from build123d import *

# Parameters (mm, degrees)
F0_W     = 32
F0_H     = 32
F1_DEPTH = 20
F2_T     = -2.5
F3_R     = 4
F4_DEPTH = 4


with BuildPart() as f1:
    # F0 (on Top) → F1 (new body)
    with BuildSketch(Plane.XY):
        with Locations((-40.726009, 25.983708)):
            Rectangle(F0_W, F0_H)
    extrude(amount=F1_DEPTH)

    # F2
    f2_openings = [f1.faces().sort_by_distance(p)[0] for p in [
        (-40.726009, 25.983708, 0),
    ]]
    offset(amount=F2_T, openings=f2_openings)

    # F3 (on face) → F4 (join)
    with BuildSketch(Plane.XY.offset(20)):
        with Locations((-49.358711, 33.123519)):
            Circle(F3_R)
        with Locations((-49.358711, 17.261552)):
            Circle(F3_R)
        with Locations((-32.003853, 17.261552)):
            Circle(F3_R)
        with Locations((-32.003853, 33.123519)):
            Circle(F3_R)
    extrude(amount=F4_DEPTH)


solid = f1.part
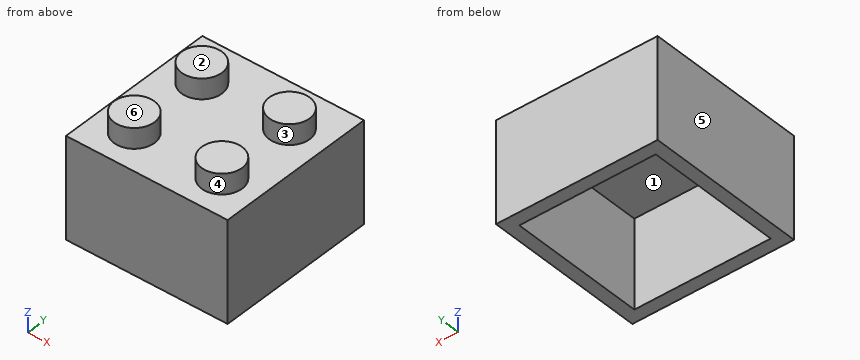
Can you work these out from the model? Positions are in its coordinate system, mm. Face numbers are marked on the shaded views. A direction names the side the tool comes from. Give positions to 0.01 mm unless a question says otherwise; leave off trailing zeros. Loops run counter-clockwise (first coordinate to the right, second up) from the corner with the lowest first, then second, coordinate; pieces in that order, holes last. Notation, with made-up numbers: M 13.25,-17.5 L 31.25,-17.5 A15 cw 31.25,4.5 Z; hole C -32.5,44.5 d11. An arc over 180 degrees is marked long. One line per item, written item: value. Start each with the question number.
1) On a 3-axis mill with a long thin cutter (end or side, diameter ignored), from which of +Z, -Z, +X, -X, +Y, -Y can I reach the whole of each face in a straight line? I mean the marked faces 1, 2 and 3. Say none if no direction works.
2) Thinking about a two-plate mould opening in X: for the marked faces 4, 5 and 6, which applies, +X half, -X half, draft (parallel to the pull), parting line (faces both ways), or undercut?
3) I'm going to push flat-ended pins straight in: pin 1 (1.5 mm diameter, centred on x = -42.5, y = 17.5, fed in from -Z); pin 2 (3 mm diameter, centred on x = -36.5, y = 21.5, fed in from +Z). Where does each tip first touch, or does it pass through?
4) If we section it at A-A, the plane z = 10.5: Write out the boundary of the cut face in (x, y), and give its area (3 significant figures).
5) If we section it at B-B, the plane x = -41: Write out the boundary of the cut face in (y, z).
6) If I drill on line 1 (X direction, y = 16, z = 7.75); line 2 (Y direction, x = -40.5, z = 9.75); line 3 (Z direction, x = -43, y = 40), over which ranges is the centre line in solid material (lowest first)? Write a range as [from, to].
7) If we section it at D-D, the plane x = -32.5: Write out the boundary of the cut face in (y, z), and give its area (3 significant figures).
8) If we section it at C-C, the plane y = 27: Write out the boundary of the cut face in (x, z).
Completed:
1. face 1: -Z
1. face 2: +Z, +X, -X, +Y, -Y
1. face 3: +Z
2. face 4: undercut
2. face 5: -X half
2. face 6: draft
3. pin 1: stops at z = 17.5
3. pin 2: stops at z = 20
4. outline: M -56.73,9.98 L -24.73,9.98 L -24.73,41.98 L -56.73,41.98 Z; hole M -54.23,12.48 L -27.23,12.48 L -27.23,39.48 L -54.23,39.48 Z
4. area: 295 mm^2
5. outline: M 9.98,0 L 12.48,0 L 12.48,17.5 L 39.48,17.5 L 39.48,0 L 41.98,0 L 41.98,20 L 9.98,20 Z
6. line 1: x = [-56.73, -54.23], [-27.23, -24.73]
6. line 2: y = [9.98, 12.48], [39.48, 41.98]
6. line 3: z = [0, 20]
7. outline: M 9.98,0 L 12.48,0 L 12.48,17.5 L 39.48,17.5 L 39.48,0 L 41.98,0 L 41.98,20 L 37.09,20 L 37.09,24 L 29.15,24 L 29.15,20 L 21.23,20 L 21.23,24 L 13.29,24 L 13.29,20 L 9.98,20 Z
7. area: 231 mm^2
8. outline: M -56.73,0 L -54.23,0 L -54.23,17.5 L -27.23,17.5 L -27.23,0 L -24.73,0 L -24.73,20 L -56.73,20 Z
